Autodesk Inventor part; units mm, degrees
ref_plane "YZ Plane" through (0, 0, 0) normal (1, 0, 0) x (0, 1, 0)
ref_plane "XZ Plane" through (0, 0, 0) normal (0, 1, 0) x (-1, 0, 0)
ref_plane "XY Plane" through (0, 0, 0) normal (0, 0, 1) x (1, 0, 0)
sketch "Sketch1" plane through (0, 0, 0) normal (0, 1, 0) x (-1, 0, 0)
  line L0 (0, 0) -> (0, -10)
  line L1 (0, -10) -> (-20, -10)
  line L2 (-20, -10) -> (-20, 0)
  line L3 (-20, 0) -> (0, 0)
  arc A0 (0, -3.3117) -> (0, -5.8117) centre (-3, -4.5617) ccw
  arc A1 (-20, -5.8117) -> (-20, -3.3117) centre (-17, -4.5617) ccw
  line L4 (-10, 0) -> (-10, -10) construction
  circle A2 centre (-3, -4.5617) radius 1.75
  circle A3 centre (-17, -4.5617) radius 1.75
  dimension "d2" = 10
  dimension "d3" = 20
  dimension "d5" = 6.5
  dimension "d8" = 7
  dimension "d9" = 7
  dimension "d11" = 3.5
  dimension "d12" = 3.5
  dimension "d13" = 10
  dimension "d14" = 3.3117
  dimension "d15" = 4.5617
extrude "Extrusion1" add sketch "Sketch1" along normal blind 1.5 contours L0 A0 | A1 L2
extrude "Extrusion2" add sketch "Sketch1" along normal blind 3 contours L0 A0 L1 L2 A1 L3
properties part number "reverse gear bearing keeper"
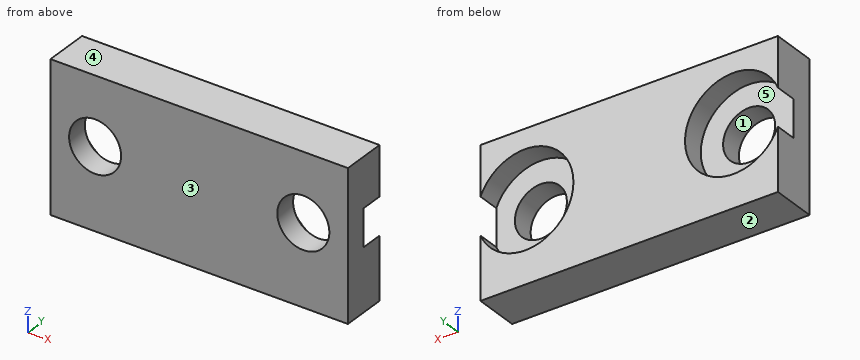
Here's how the part is built. I have some questions about the finished solid (model axes, mm). Face numbers are marked on the shaded views. A direction names the side the tool comes from. Coordinates: 2 decimals unless noted, no trailing zeros. Order: outer loops, then holes, each group sorted by start corner. A loop starts at its lowest first (then second) coordinate and runs counter-clockwise, first axis right, second up.
Item 1: If we section it at A-A on z = -4.75: List the corners of the cut face in (x, y) for me, plus the area to 3 significant figures.
Result sheet:
outline: (0, 0) - (1.26, 0) - (1.26, 1.5) - (0, 1.5) - close; (4.74, 0) - (15.26, 0) - (15.26, 1.5) - (13.76, 1.5) - (13.76, 3) - (6.24, 3) - (6.24, 1.5) - (4.74, 1.5) - close; (18.74, 0) - (20, 0) - (20, 1.5) - (18.74, 1.5) - close
area: 30.8 mm2
Item 2: For the marked faces 4 and 5, which set-ups out of +Z, -Z, +X, -X, +Y, -Y let a thin tool reach every point of the face, with its end or its side?
Result sheet:
face 4: +Z, +X, -X, +Y, -Y
face 5: +Y
Item 3: If we mould it in two halves opening along Z, with no side actions, what happens to the marked faces 1, 2 and 3? For each: +Z half, -Z half, draft (parallel to the pull), parting line (faces both ways), or undercut.
Result sheet:
face 1: undercut
face 2: -Z half
face 3: draft
Item 4: For P1, Ø5, axis at x = 16.5, z = -4.5, coming from the +Y side, with a flat end and sliding along its axis, tell me the tip position at first contact or that it passes through.
Result sheet:
P1: stops at y = 1.5
Item 5: If we section it at C-C on y = 0.9: List the corners of the cut face in (x, z) for me, plus the area to 3 significant figures.
Result sheet:
outline: (0, -10) - (20, -10) - (20, 0) - (0, 0) - close; hole circle Ø3.5 at (3, -4.56); hole circle Ø3.5 at (17, -4.56)
area: 181 mm2
Item 6: If we section it at D-D on z = -2: List the corners of the cut face in (x, y) for me.
Result sheet:
outline: (0, 0) - (20, 0) - (20, 3) - (19, 3) - (19, 1.5) - (15, 1.5) - (15, 3) - (5, 3) - (5, 1.5) - (1, 1.5) - (1, 3) - (0, 3) - close
Item 7: I need wall thicknesses on line 1 (Z direction, x = 17, y = 1.9); line 2 (X direction, y = 1.6, z = -2); line 3 (X direction, y = 1.4, z = -3.5). Which ranges of each line are inside material? Lowest first, please.
Result sheet:
line 1: z = -10 to -7.81, -1.31 to 0
line 2: x = 0 to 1, 5 to 15, 19 to 20
line 3: x = 0 to 1.61, 4.39 to 15.61, 18.39 to 20
Item 8: If we section it at B-B on x = 17: List the corners of the cut face in (y, z) for me.
Result sheet:
outline: (0, -10) - (3, -10) - (3, -7.81) - (1.5, -7.81) - (1.5, -6.31) - (0, -6.31) - close; (0, -2.81) - (1.5, -2.81) - (1.5, -1.31) - (3, -1.31) - (3, 0) - (0, 0) - close
